```python
from build123d import *

# Parameters (mm, degrees)
SKETCH1_W           = 2
SKETCH1_H           = 7
SKETCH1_R           = 2
BOSS_EXTRUDE1_DEPTH = 2
SKETCH2_W           = 23.15
SKETCH2_H           = 50
CUT_EXTRUDE1_DEPTH  = 10


with BuildPart() as part:
    # Sketch1 → Boss-Extrude1 (new body)
    with BuildSketch(Plane(origin=(0, 0, 0), x_dir=(1, 0, 0), z_dir=(0, 1, 0))):
        Polygon((-47.649453113, 2.019339096), (-70.799453113, 2.019339096), (-70.799453113, -47.980660904), (-47.649453113, -47.980660904), (-47.649453113, -45.980660904), (-42.649453113, -45.980660904), (-42.649453113, -47.980660904), (4.050546887, -47.980660904), (4.050546887, -45.980660904), (9.050546887, -45.980660904), (9.050546887, -47.980660904), (32.200546887, -47.980660904), (32.200546887, 2.019339096), (9.050546887, 2.019339096), (9.050546887, 0.019339096), (4.050546887, 0.019339096), (4.050546887, 2.019339096), (-42.649453113, 2.019339096), (-42.649453113, 0.019339096), (-47.649453113, 0.019339096), align=None)
        with Locations((-36.649453113, -38.480660904)):
            Rectangle(SKETCH1_W, SKETCH1_H, mode=Mode.SUBTRACT)
        with Locations((-1.949453113, -38.480660904)):
            Rectangle(SKETCH1_W, SKETCH1_H, mode=Mode.SUBTRACT)
        with Locations(Location((-19.299453113, -32.980660904, 0), (0, 0, 270))):
            Circle(SKETCH1_R, mode=Mode.SUBTRACT)
        with Locations((-36.649453113, -22.980660904)):
            Rectangle(SKETCH1_W, SKETCH1_H, mode=Mode.SUBTRACT)
        with Locations(Location((-42.649453113, -12.980660904, 0), (0, 0, 270))):
            Circle(SKETCH1_R, mode=Mode.SUBTRACT)
        with Locations((-36.649453113, -7.480660904)):
            Rectangle(SKETCH1_W, SKETCH1_H, mode=Mode.SUBTRACT)
        with Locations((-1.949453113, -22.980660904)):
            Rectangle(SKETCH1_W, SKETCH1_H, mode=Mode.SUBTRACT)
        with Locations(Location((4.050546887, -12.980660904, 0), (0, 0, 270))):
            Circle(SKETCH1_R, mode=Mode.SUBTRACT)
        with Locations((-1.949453113, -7.480660904)):
            Rectangle(SKETCH1_W, SKETCH1_H, mode=Mode.SUBTRACT)
    extrude(amount=BOSS_EXTRUDE1_DEPTH)

    # Sketch2 → Cut-Extrude1 (cut)
    with BuildSketch(Plane(origin=(0, 0, 0), x_dir=(-1, 0, 0), z_dir=(0, -1, 0))):
        with Locations((59.224453113, -22.980660904)):
            Rectangle(SKETCH2_W, SKETCH2_H)
        with Locations((-20.625546887, -22.980660904)):
            Rectangle(SKETCH2_W, SKETCH2_H)
    extrude(amount=-CUT_EXTRUDE1_DEPTH, mode=Mode.SUBTRACT)


solid = part.part
```
Geometry: final body of the model. Coordinates: model frame, mm. A direction names the side the tool comes from. Round coordinates to 2 decimals unless told otherwise and drop trailing zeros. Order: outer loops, then holes, each group sorted by start corner. A loop starts at its lowest first (then second) coordinate and runs counter-clockwise, first axis right, second up. Notation, with made-up numbers: M 8,72 L 46,72 A16 cw 46,102 Z; hole C -30,28.25 d9. An arc over 180 degrees is marked long. Use one line per item in the form item = value. Start each with the question number.
Q1. Cut plane C-C (y = 1.3). Count the separate pieces of the cut face and the enclosed holes in it, and give its area (3 significant figures).
Q2. Mould query, pull axis X, two halves, no side actions, for faces 5 (the face through (-42.649, 1, -1)), 6 (the face through (-20, 2, 23)), 7 (the face through (-2, 1, 10.981)). Classes: +X half, -X half, draft (parallel to the pull), parting line (faces both ways), or undercut.
Q3. Cut plane B-B (z = 39). Return loops of the section in (x, y), and give its area (3 significant figures).
Q4. Material intervals for line 1 (X direction, y = 1.55, z = 21.5); line 2 (X direction, y = 1.35, z = 13); line 3 (Z direction, x = -19.5, y = 1.4), sorted ascending. Write a range as [from, to].
Q5. Access query for faces 1 (the face through (-37, 1, 41.981)), 2 (the face through (-45, 1, 45.981)), 3 (the face through (-20, 0, 23)), 4 (the face through (4.051, 1, 47)). Directions: +Z, -Z, +X, -X, +Y, -Y. A direction counts if a zero-diameter tool reaches every point of the face in a straight line with its end or side. Return the directions, or none.
Q6. Pin query (flat end, axial travel): pin 1 Ø2.5 at (x, z) = (4.05, 12.98) entering from -Y. Return the tip coordinate at first contact, or that it passes through.
Q7. Cut plane A-A (x = -2). Return loops of the section in (y, z), and give its area (3 significant figures).
Geometry results:
q1.separate_pieces = 1
q1.enclosed_holes = 9
q1.area = 2,670 mm^2
q2.face_5 = -X half
q2.face_6 = draft
q2.face_7 = undercut
q3.outline = M -47.65,0 L -37.65,0 L -37.65,2 L -47.65,2 Z; M -35.65,0 L -2.95,0 L -2.95,2 L -35.65,2 Z; M -0.95,0 L 9.05,0 L 9.05,2 L -0.95,2 Z
q3.area = 105 mm^2
q4.line_1 = [-47.65, -37.65], [-35.65, -2.95], [-0.95, 9.05]
q4.line_2 = [-47.65, -44.65], [-40.65, 2.05], [6.05, 9.05]
q4.line_3 = [-2.02, 30.99], [34.97, 47.98]
q5.face_1 = +Y, -Y
q5.face_2 = +Z, -X, +Y, -Y
q5.face_3 = +Z, -Z, +X, -X, -Y
q5.face_4 = +Z, +X, +Y, -Y
q6.pin_1 = through
q7.outline = M 0,-2.02 L 2,-2.02 L 2,3.98 L 0,3.98 Z; M 0,10.98 L 2,10.98 L 2,19.48 L 0,19.48 Z; M 0,26.48 L 2,26.48 L 2,34.98 L 0,34.98 Z; M 0,41.98 L 2,41.98 L 2,47.98 L 0,47.98 Z
q7.area = 58.0 mm^2
